Geometry: final body of the model. Coordinates: model frame, mm. A direction names the side the tool comes from. Give positions to 0.01 mm unless a question says otherwise; leave off trailing zeros. Order: outer loops, then holes, each group sorted by start corner. A loop starts at its lowest first (then second) coordinate and runs counter-clockwise, first axis right, second up. Notation, with made-up numbers: (-9.5, 7.25) -> (19.5, 7.25) arc R26 ccw to (19.5, 31.25) -> close; hole circle Ø1 at (39.25, 42.5). An arc over 180 degrees is marked (long way). Answer in a Markdown table with one row per item. Add a question column.
Q1. Line query: line 1 along X through (y, z) = (-15.5, 10.75); line 2 along X through (y, z) = (15, 28); line 3 along Y through (x, z) = (-15, 23). Output: solid intervals per line, ascending. Write a range as from..to.
Q2. Set-up query: faces 4 (the face through (15, -15, 30)), 5 (the face through (7.5, -25, 7)), 6 (the face through (-7.5, -25, 7)), 7 (the face through (10, 35, 44)). Return all of +Z, -Z, +X, -X, +Y, -Y with unobstructed straight access to the full face (end or side cutting, diameter ignored); none if empty.
Q3. Cut plane D-D on y = -15.5. Return the cut outline in (x, z).
Q4. Contact query for flat-ended pins moving along their axis: P1, Ø12, axis at x = -2.5, y = -20, coming from the -Z side; P2, Ø6, axis at x = -1.5, z = 40, coming from the -Y side; P3, Ø3.5, axis at y = 42.5, z = 45, coming from the +X side; P4, Ø3.5, axis at y = 37, z = 43.5, coming from the -X side. Output: stop coordinate, or through.
Q5. Cut plane C-C on x = -5. Return the cut outline in (y, z).
Q6. Cut plane B-B on x = -15.5. Return the cut outline in (y, z), and give its area (3 significant figures).
Q7. Cut plane A-A on z = 21. Return the cut outline in (x, y), and give its area (3 significant figures).
Q8. Pull-direction query (Y, two-part tool) for faces 1 (the face through (-16, 16, 30)), 2 (the face through (19.7, 19.8, 14.8)), 3 (the face through (-20, 20, 30)); classes: +Y half, -Y half, draft (parallel to the pull), parting line (faces both ways), or undercut.
from build123d import *

# Parameters (mm, degrees)
F0_W      = 42
F0_H      = 42
F1_DEPTH  = 30
F2_SIZE   = 2.5
F3_R      = 1.5
F4_DEPTH  = 10
F5_R      = 11
F6_DEPTH  = 2
F8_DEPTH  = 24
F9_W      = 15
F9_H      = 5
F10_DEPTH = 7.5
F12_DEPTH = 38.1
F13_R     = 3
F14_DEPTH = 7.5
F15_W     = 20
F15_H     = 11.25
F16_DEPTH = 12.7
F18_DEPTH = 8
F19_SIZE  = 3.5
F20_R     = 2
F21_DEPTH = 25


with BuildPart() as f1:
    # F0 (on Top) → F1 (new body)
    with BuildSketch(Plane.XY):
        Rectangle(F0_W, F0_H)
    extrude(amount=F1_DEPTH)

    # F2
    f2_edges = [f1.edges().sort_by_distance(p)[0] for p in [
        (-21, -21, 15),
        (21, -21, 15),
        (21, 21, 15),
        (-21, 21, 15),
    ]]
    chamfer(f2_edges, length=F2_SIZE)

    # F3 (on face) → F4 (cut)
    with BuildSketch(Plane.XY.offset(30)):
        with Locations((-15.5, 15.5)):
            Circle(F3_R)
        with Locations((15.5, 15.5)):
            Circle(F3_R)
        with Locations((15.5, -15.5)):
            Circle(F3_R)
        with Locations((-15.5, -15.5)):
            Circle(F3_R)
    extrude(amount=-F4_DEPTH, mode=Mode.SUBTRACT)

    # F5 (on face) → F6 (join)
    with BuildSketch(Plane.XY.offset(30)):
        Circle(F5_R)
    extrude(amount=F6_DEPTH)

    # F7 (on face) → F8 (join)
    with BuildSketch(Plane.XY.offset(32)):
        with BuildLine():
            Line((2.193171, 1.2), (-2.193171, 1.2))
            ThreePointArc((-2.193171, 1.2), (0, -2.5), (2.193171, 1.2))
        make_face()
    extrude(amount=F8_DEPTH)

    # F9 (on face) → F10 (join)
    with BuildSketch(Plane.XZ.offset(21)):
        with Locations((0, 7.5)):
            Rectangle(F9_W, F9_H)
    extrude(amount=F10_DEPTH)

    # F11 (on face) → F12 (join)
    with BuildSketch(Plane.XY.offset(30)):
        with BuildLine():
            Line((-18.5, -21), (18.5, -21))
            ThreePointArc((18.5, -21), (20.267767, -20.267767), (21, -18.5))
            Line((21, -18.5), (21, 18.5))
            ThreePointArc((21, 18.5), (20.267767, 20.267767), (18.5, 21))
            Line((18.5, 21), (-18.5, 21))
            ThreePointArc((-18.5, 21), (-20.267767, 20.267767), (-21, 18.5))
            Line((-21, 18.5), (-21, -18.5))
            ThreePointArc((-21, -18.5), (-20.267767, -20.267767), (-18.5, -21))
        make_face()
    extrude(amount=F12_DEPTH)

    # F13 (on face) → F14 (join)
    with BuildSketch(Plane(origin=(0, 21, 0), x_dir=(-1, 0, 0), z_dir=(0, 1, 0))):
        with Locations((0, 44.475)):
            Circle(F13_R)
    extrude(amount=F14_DEPTH)

    # F15 (on face) → F16 (join)
    with BuildSketch(Plane(origin=(0, 28.5, 0), x_dir=(-1, 0, 0), z_dir=(0, 1, 0))):
        with Locations((0, 44.475)):
            Rectangle(F15_W, F15_H)
    extrude(amount=F16_DEPTH)

    # F17 (on face) → F18 (join)
    with BuildSketch(Plane(origin=(0, 41.2, 0), x_dir=(-1, 0, 0), z_dir=(0, 1, 0))):
        Polygon((3.75, 42.309936), (3.75, 46.640064), (0, 48.805127), (-3.75, 46.640064), (-3.75, 42.309936), (0, 40.144873), align=None)
    extrude(amount=F18_DEPTH)

    # F19
    f19_edges = [f1.edges().sort_by_distance(p)[0] for p in [
        (-1.875, 49.2, 41.227405),
        (1.875, 49.2, 47.722595),
        (-3.75, 49.2, 44.475),
        (1.875, 49.2, 41.227405),
        (3.75, 49.2, 44.475),
        (-1.875, 49.2, 47.722595),
    ]]
    chamfer(f19_edges, length=F19_SIZE)

    # F20 (on face) → F21 (cut)
    with BuildSketch(Plane(origin=(0, 0, 0), x_dir=(1, 0, 0), z_dir=(0, 0, -1))):
        with Locations((-15.5, 15.5)):
            Circle(F20_R)
        with Locations((15.5, 15.5)):
            Circle(F20_R)
    extrude(amount=-F21_DEPTH, mode=Mode.SUBTRACT)


solid = f1.part
Completed:
| question | item | result |
|---|---|---|
| 1 | line 1 | x = -21..-17.5, -13.5..13.5, 17.5..21 |
| 1 | line 2 | x = -21..-16.91, -14.09..14.09, 16.91..21 |
| 1 | line 3 | y = -21..-17.44, -13.56..14.09, 16.91..21 |
| 2 | face 4 | -Z |
| 2 | face 5 | +Z, -Z, +X, -Y |
| 2 | face 6 | +Z, -Z, -X, -Y |
| 2 | face 7 | +Z, -Z, +X, +Y |
| 3 | outline | (-21, 0) -> (-17.5, 0) -> (-17.5, 25) -> (-17, 25) -> (-17, 30) -> (-14, 30) -> (-14, 25) -> (-13.5, 25) -> (-13.5, 0) -> (13.5, 0) -> (13.5, 25) -> (14, 25) -> (14, 30) -> (17, 30) -> (17, 25) -> (17.5, 25) -> (17.5, 0) -> (21, 0) -> (21, 68.1) -> (-21, 68.1) -> close |
| 4 | P1 | stops at z = 0 |
| 4 | P2 | stops at y = -21 |
| 4 | P3 | stops at x = 10 |
| 4 | P4 | stops at x = -10 |
| 5 | outline | (-28.5, 5) -> (-21, 5) -> (-21, 0) -> (21, 0) -> (21, 68.1) -> (-21, 68.1) -> (-21, 10) -> (-28.5, 10) -> close; (28.5, 38.85) -> (41.2, 38.85) -> (41.2, 50.1) -> (28.5, 50.1) -> close |
| 6 | outline | (-21, 0) -> (-17.5, 0) -> (-17.5, 25) -> (-17, 25) -> (-17, 30) -> (-14, 30) -> (-14, 25) -> (-13.5, 25) -> (-13.5, 0) -> (21, 0) -> (21, 68.1) -> (-21, 68.1) -> close; hole (14, 20) -> (17, 20) -> (17, 30) -> (14, 30) -> close |
| 6 | area | 2,720 mm² |
| 7 | outline | (-21, -18.5) -> (-18.5, -21) -> (18.5, -21) -> (21, -18.5) -> (21, 18.5) -> (18.5, 21) -> (-18.5, 21) -> (-21, 18.5) -> close; hole circle Ø4 at (-15.5, -15.5); hole circle Ø3 at (-15.5, 15.5); hole circle Ø4 at (15.5, -15.5); hole circle Ø3 at (15.5, 15.5) |
| 7 | area | 1,710 mm² |
| 8 | face 1 | undercut |
| 8 | face 2 | +Y half |
| 8 | face 3 | draft |
